Autodesk Inventor part; units mm, degrees
ref_plane "YZ Plane" through (0, 0, 0) normal (1, 0, 0) x (0, 1, 0)
ref_plane "XZ Plane" through (0, 0, 0) normal (0, 1, 0) x (-1, 0, 0)
ref_plane "XY Plane" through (0, 0, 0) normal (0, 0, 1) x (1, 0, 0)
sketch "Sketch1" plane through (0, 0, 0) normal (0, 0, 1) x (1, 0, 0)
  circle A0 centre (-86.5, 0) radius 11
  circle A1 centre (86.5, 0) radius 11
  circle A2 centre (-75, 44.5) radius 5.5
  circle A3 centre (-75, -44.5) radius 5.5
  circle A4 centre (75, 44.5) radius 5.5
  circle A5 centre (75, -44.5) radius 5.5
  circle A6 centre (-65.5, 0) radius 3
  circle A7 centre (65.5, 0) radius 3
  circle A8 centre (-44.5, 44.5) radius 4.1881
  circle A9 centre (-44.5, -44.5) radius 4.1881
  circle A10 centre (44.5, 44.5) radius 4.1881
  circle A11 centre (44.5, -44.5) radius 4.1881
  line L0 (100, -58) -> (98, -60) construction
  line L1 (100, 58) -> (100, -58) construction
  line L2 (98, 60) -> (100, 58) construction
  line L3 (-98, 60) -> (98, 60)
  line L4 (-100, 58) -> (-98, 60) construction
  line L5 (-100, -58) -> (-100, 58) construction
  line L6 (-98, -60) -> (-100, -58) construction
  line L7 (98, -60) -> (-98, -60)
  line L8 (98, 60) -> (119, 60)
  line L9 (122, 57) -> (122, -57)
  line L10 (119, -60) -> (98, -60)
  line L11 (98, -60) -> (98, 60) construction
  line L12 (-98, 60) -> (-119, 60)
  line L13 (-122, 57) -> (-122, -57)
  line L14 (-119, -60) -> (-98, -60)
  line L15 (-98, -60) -> (-98, 60) construction
  line L16 (119, 60) -> (122, 57)
  line L17 (119, -60) -> (122, -57)
  line L18 (-122, -57) -> (-119, -60)
  line L19 (-122, 57) -> (-119, 60)
  point P0 (0, 0)
  point P1 (122, -60)
  point P2 (122, 60)
  point P3 (-122, -60)
  point P4 (-122, 60)
  dimension "d4" = 3
  dimension "d5" = 3
  dimension "d6" = 3
  dimension "d7" = 3
  dimension "d8" = 3
  dimension "d9" = 3
  dimension "d10" = 3
  dimension "d11" = 3
  dimension "d12" = 22
  dimension "d13" = 22
extrude "Extrusion1" add sketch "Sketch1" along normal blind 10
equation "\"d13\" = d12"
properties part number "TilesGrip"
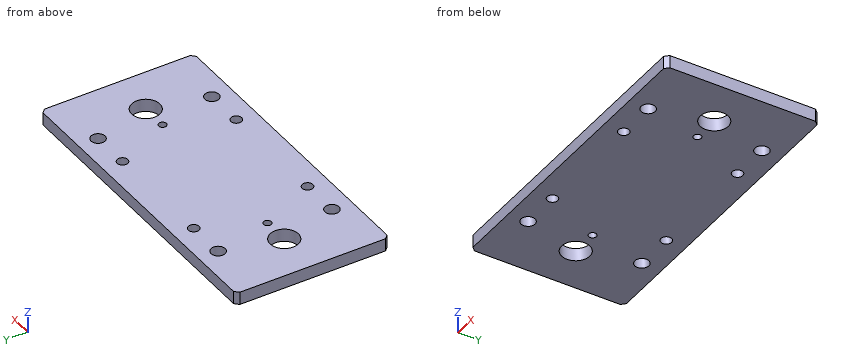
Source: CAD feature listing. Evaluate the final solid. Frame: model axes, mm. Give positions to 0.01 mm unless a question says otherwise; leave off trailing zeros. Write each loop counter-clockwise with the first axis right and the second up, starting at its lowest first coordinate (ties: lowest second). Pieces come first, ordered by that corner, then holes. Notation, with made-up numbers: (9, 30) -> (56, 30) arc R25 ccw to (56, 47) -> close; hole circle Ø4 at (89, -3.5). An arc over 180 degrees is marked (long way). Return JSON: item names as keys, results as strings. Group by question number.
1. Section C-C, the plane y = 0. Output: boundary loops of the cut face in (x, z).
2. Material intervals for line 1 (Y direction, x = -44.5, z = 7.25); line 2 (X direction, y = 46, z = 9.25); line 3 (X direction, y = -42, z = 8.25), sorted ascending. Write a range as from..to.
3. Section B-B, the plane z = 4.25. Count the separate pieces of the cut face and the enclosed holes in it, then the cut area to 3 significant figures.
4. Section D-D, the plane x = 44.5. Output: boundary loops of the cut face in (y, z), then the cut area to 3 significant figures.
5. Section A-A, the plane x = 86.5. Output: boundary loops of the cut face in (y, z).
Determined:
{
 "1": {"outline": "(-122, 0) -> (-97.5, 0) -> (-97.5, 10) -> (-122, 10) -> close; (-75.5, 0) -> (-68.5, 0) -> (-68.5, 10) -> (-75.5, 10) -> close; (-62.5, 0) -> (62.5, 0) -> (62.5, 10) -> (-62.5, 10) -> close; (68.5, 0) -> (75.5, 0) -> (75.5, 10) -> (68.5, 10) -> close; (97.5, 0) -> (122, 0) -> (122, 10) -> (97.5, 10) -> close"},
 "2": {"line 1": "y = -60..-48.69, -40.31..40.31, 48.69..60", "line 2": "x = -122..-80.29, -69.71..-48.41, -40.59..40.59, 48.41..69.71, 80.29..122", "line 3": "x = -122..-79.9, -70.1..-47.86, -41.14..41.14, 47.86..70.1, 79.9..122"},
 "3": {"separate pieces": "1", "enclosed holes": "12", "area": "27,800 mm2"},
 "4": {"outline": "(-60, 0) -> (-48.69, 0) -> (-48.69, 10) -> (-60, 10) -> close; (-40.31, 0) -> (40.31, 0) -> (40.31, 10) -> (-40.31, 10) -> close; (48.69, 0) -> (60, 0) -> (60, 10) -> (48.69, 10) -> close", "area": "1,030 mm2"},
 "5": {"outline": "(-60, 0) -> (-11, 0) -> (-11, 10) -> (-60, 10) -> close; (11, 0) -> (60, 0) -> (60, 10) -> (11, 10) -> close"}
}
